Check sheet for the modelled part. Datum: model origin and axes. Units: mm. A direction names the side the tool comes from. Give positions to 0.01 mm unless a question says otherwise; leave off trailing zeros. Order: outer loops, then holes, each group sorted by start corner. A loop starts at its lowest first (then second) coordinate and runs counter-clockwise, first axis right, second up.
```python
from build123d import *

# Parameters (mm, degrees)
F1_DEPTH  = 3
F3_D      = 7
F4_W      = 24
F4_H      = 24.5219291974
F5_DEPTH  = 27
F6_R      = 1.55
F7_DEPTH  = 12.5
F8_R      = 1.75
F9_DEPTH  = 12
F10_R     = 4
F11_DEPTH = 3.4
F12_R     = 7
F13_R     = 7
F14_R     = 7
F15_R     = 7
F16_W     = 1
F16_H     = 6
F17_DEPTH = 14
F18_R     = 5
F19_DEPTH = 15
F20_R     = 3
F20_R_2   = 1.55
F21_DEPTH = 3


with BuildPart() as f1:
    # F0 (on Top) → F1 (new body)
    with BuildSketch(Plane.XY):
        with BuildLine():
            Line((42.5, 5), (42.5, -5))
            Line((42.5, -5), (36.1522351233, -5))
            ThreePointArc((36.1522351233, -5), (45.1458596679, -7.635020992), (50.5804776424, 0))
            ThreePointArc((50.5804776424, 0), (45.1458596679, 7.635020992), (36.1522351233, 5))
            Line((36.1522351233, 5), (42.5, 5))
        make_face()
        with BuildLine():
            ThreePointArc((-36.1522351233, 5), (-50.5804776424, 0), (-36.1522351233, -5))
            Line((-36.1522351233, -5), (-42.5, -5))
            Line((-42.5, -5), (-42.5, 5))
            Line((-42.5, 5), (-36.1522351233, 5))
        make_face()
        with BuildLine():
            Line((36.1522351233, -5), (42.5, -5))
            Line((42.5, -5), (42.5, 5))
            Line((42.5, 5), (36.1522351233, 5))
            ThreePointArc((36.1522351233, 5), (34.4195223576, 0), (36.1522351233, -5))
        make_face()
        with BuildLine():
            Line((-36.1522351233, -5), (36.1522351233, -5))
            ThreePointArc((36.1522351233, -5), (34.4195223576, 0), (36.1522351233, 5))
            Line((36.1522351233, 5), (-36.1522351233, 5))
            ThreePointArc((-36.1522351233, 5), (-34.864979008, 2.6458596679), (-34.4195223576, 0))
            ThreePointArc((-34.4195223576, 0), (-34.864979008, -2.6458596679), (-36.1522351233, -5))
        make_face()
        with BuildLine():
            Line((-42.5, -5), (-36.1522351233, -5))
            ThreePointArc((-36.1522351233, -5), (-34.864979008, -2.6458596679), (-34.4195223576, 0))
            ThreePointArc((-34.4195223576, 0), (-34.864979008, 2.6458596679), (-36.1522351233, 5))
            Line((-36.1522351233, 5), (-42.5, 5))
            Line((-42.5, 5), (-42.5, -5))
        make_face()
    extrude(amount=F1_DEPTH)

    # F3 (through all)
    with Locations(Plane.XY.offset(3)):
        with Locations((-42.5, 0), (42.5, 0)):
            Hole(F3_D / 2)

    # F4 (on Top) → F5 (join)
    with BuildSketch(Plane.XY):
        Rectangle(F4_W, F4_H)
    extrude(amount=F5_DEPTH)

    # F6 (on Front) → F7 (cut, symmetric)
    with BuildSketch(Plane.XZ):
        with Locations((0, 21.0996698588)):
            Circle(F6_R)
    extrude(amount=F7_DEPTH, both=True, mode=Mode.SUBTRACT)

    # F8 (on face) → F9 (cut)
    with BuildSketch(Plane(origin=(-12, 0, 0), x_dir=(0, -1, 0), z_dir=(-1, 0, 0))):
        with Locations((0, 21.061129868)):
            Circle(F8_R)
    extrude(amount=-F9_DEPTH, mode=Mode.SUBTRACT)

    # F10 (on face) → F11 (cut)
    with BuildSketch(Plane(origin=(-12, 0, 0), x_dir=(0, -1, 0), z_dir=(-1, 0, 0))):
        with Locations((0, 21.061129868)):
            Circle(F10_R)
    extrude(amount=-F11_DEPTH, mode=Mode.SUBTRACT)

    # F12
    f12_edges = [f1.edges().sort_by_distance(p)[0] for p in [
        (-12, 12.260965, 13.5),
    ]]
    fillet(f12_edges, radius=F12_R)

    # F13
    f13_edges = [f1.edges().sort_by_distance(p)[0] for p in [
        (12, 12.260965, 13.5),
    ]]
    fillet(f13_edges, radius=F13_R)

    # F14
    f14_edges = [f1.edges().sort_by_distance(p)[0] for p in [
        (-12, -12.260965, 13.5),
    ]]
    fillet(f14_edges, radius=F14_R)

    # F15
    f15_edges = [f1.edges().sort_by_distance(p)[0] for p in [
        (12, -12.260965, 13.5),
    ]]
    fillet(f15_edges, radius=F15_R)

    # F16 (on face) → F17 (cut)
    with BuildSketch(Plane.XY.offset(27)):
        Rectangle(F16_W, F16_H)
    extrude(amount=-F17_DEPTH, mode=Mode.SUBTRACT)

    # F18 (on face) → F19 (cut)
    with BuildSketch(Plane(origin=(0, 0, 0), x_dir=(1, 0, 0), z_dir=(0, 0, -1))):
        Circle(F18_R)
    extrude(amount=-F19_DEPTH, mode=Mode.SUBTRACT)

    # F20 (on face) → F21 (cut)
    with BuildSketch(Plane(origin=(0, 12.2609645987, 0), x_dir=(-1, 0, 0), z_dir=(0, 1, 0))):
        with Locations((0, 21.0996698588)):
            Circle(F20_R)
        with Locations((0, 21.0996698588)):
            Circle(F20_R_2, mode=Mode.SUBTRACT)
    extrude(amount=-F21_DEPTH, mode=Mode.SUBTRACT)


solid = f1.part
```
(1) Cross-section at A-A on x = -42.5. Enter the section's corners in (y, z).
Response values:
outline: (-8.08, 0) - (-3.5, 0) - (-3.5, 3) - (-8.08, 3) - close; (3.5, 0) - (8.08, 0) - (8.08, 3) - (3.5, 3) - close
(2) Gauge pin test, flat ends, axial feed: pin 1 Ø6 at (y, z) = (-5.5, 3) entering from -X; pin 2 Ø4 at (y, z) = (0, 21) entering from -X; pin 3 Ø0.9 at (x, z) = (30, 2) entering from +Y; pin 4 Ø4 at (x, y) = (42.5, 0) entering from +Z. Record the tip position at first contact, or that the pin passes through.
Response values:
pin 1: stops at x = -50.18
pin 2: stops at x = -8.6
pin 3: stops at y = 5
pin 4: passes through
(3) Set-up check for faces 4 (the face through (-4.607, -1.617, 20.391)), 5 (the face through (-1.08, 4.88, 7.4)), 6 (the face through (24, 5, 1)): record each of +Z, -Z, +X, -X, +Y, -Y from which the full face is reachable in a straight line by a thin tool's end or side.
Response values:
face 4: -X
face 5: -Z
face 6: +Z, -Z, +Y
(4) Release check for a two-part mould opening along X. For faces 1 (the face through (46, 0, 1)), 2 (the face through (-1, 6, 0)), 3 (the face through (-8.6, -2, 20)) record: released by +X, released by -X, zero draft, split by the parting line, or undercut.
Response values:
face 1: undercut
face 2: zero draft
face 3: released by -X
(5) Cross-section at D-D on x = -31. Enter the section's corners in (y, z), then the cut area to 3 significant figures.
Response values:
outline: (-5, 0) - (5, 0) - (5, 3) - (-5, 3) - close
area: 30.0 mm2
(6) Material ranges on L1, parallel to X at y = 2, z = 17.25; L2, parallel to Z at x = -0.5, y = 8.25; L3, parallel to Z at x = -2.5, y = 0, recorded low to high.
Response values:
L1: x = -12 to -0.5, 0.5 to 12
L2: z = 0 to 19.63, 22.57 to 27
L3: z = 15 to 19.31, 22.81 to 27
(7) Cross-section at C-C on y = 10.5. Enter the section's corners in (x, z).
Response values:
outline: (-9.64, 0) - (9.64, 0) - (9.64, 27) - (-9.64, 27) - close; hole circle Ø6 at (0, 21.1)
(8) Cross-section at B-B on z = 9.5. Enter the section's corners in (x, y), then the cut area to 3 significant figures.
Response values:
outline: (-12, -5.26) arc R7 ccw to (-5, -12.26) - (5, -12.26) arc R7 ccw to (12, -5.26) - (12, 5.26) arc R7 ccw to (5, 12.26) - (-5, 12.26) arc R7 ccw to (-12, 5.26) - close; hole circle Ø10 at (0, 0)
area: 468 mm2
